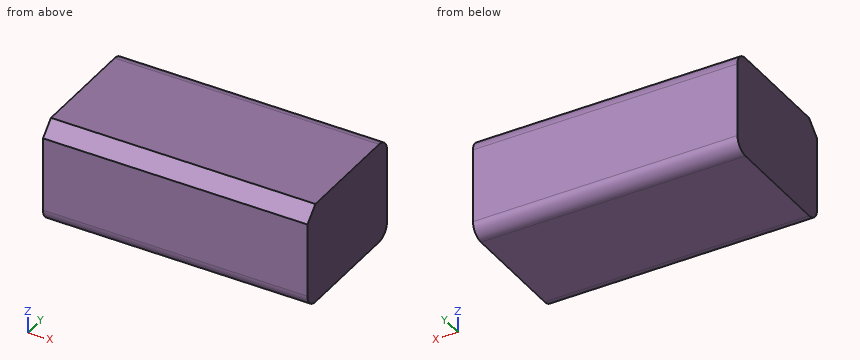
```python
from build123d import *

# Parameters (mm, degrees)
F0_W     = 99.553153
F0_H     = 38.084091
F1_DEPTH = 50.8
F2_SIZE  = 5.08
F3_R     = 5.08
F4_R     = 5.08


with BuildPart() as f1:
    # F0 (on Front) → F1 (new body)
    with BuildSketch(Plane.XZ):
        with Locations((4.676994, -4.509959)):
            Rectangle(F0_W, F0_H)
    extrude(amount=F1_DEPTH)

    # F2
    f2_edges = [f1.edges().sort_by_distance(p)[0] for p in [
        (4.676994, -50.8, 14.532087),
    ]]
    chamfer(f2_edges, length=F2_SIZE)

    # F3
    f3_edges = [f1.edges().sort_by_distance(p)[0] for p in [
        (4.676994, 0, 14.532087),
    ]]
    fillet(f3_edges, radius=F3_R)

    # F4
    f4_edges = [f1.edges().sort_by_distance(p)[0] for p in [
        (4.676994, 0, -23.552004),
        (4.676994, -50.8, -23.552004),
    ]]
    fillet(f4_edges, radius=F4_R)


solid = f1.part
```
Model file for the job. Use its own axes, mm. Coordinates: 2 decimals unless noted, no trailing zeros. Order: outer loops, then holes, each group sorted by start corner. A loop starts at its lowest first (then second) coordinate and runs counter-clockwise, first axis right, second up. Notation, with made-up numbers: (89, 22.5) - (122, 22.5) arc R19 ccw to (122, 31.5) - close; hole circle Ø4 at (40.5, -36.5). An arc over 180 degrees is marked (long way). Return JSON: item names as keys, results as strings. Group by question number.
1) Probe line 1 (Y direction, x = 39, z = 13.5); line 2 (Y direction, x = 14.5, z = -19); line 3 (Z direction, x = 30.5, y = -47.5). List the from-to ranges inside material, lowest first. Write a range as from..to.
2) Saw through at B-B, the plane y = -47. Write the cut outline in (x, z).
3) Saw through at A-A, the plane x = 5.5. Write the cut outline in (y, z).
Values found:
{
 "1": {"line 1": "y = -46.75..-2.01", "line 2": "y = -50.77..-0.03", "line 3": "z = -23.23..12.75"},
 "2": {"outline": "(-45.1, -23.39) - (54.45, -23.39) - (54.45, 13.25) - (-45.1, 13.25) - close"},
 "3": {"outline": "(-50.8, -18.47) arc R5.08 ccw to (-45.72, -23.55) - (-5.08, -23.55) arc R5.08 ccw to (0, -18.47) - (0, 9.45) arc R5.08 ccw to (-5.08, 14.53) - (-45.72, 14.53) - (-50.8, 9.45) - close"}
}
